The model under review builds one solid part; all positions refer to its coordinate system, in mm. A direction names the side the tool comes from. Give positions to 0.01 mm unless a question says otherwise; leave off trailing zeros. Order: outer loops, then holes, each group sorted by start corner. A loop starts at its lowest first (then second) coordinate and runs counter-clockwise, first axis right, second up.
```python
from build123d import *

# Parameters (mm, degrees)
SKETCH_1_W      = 69.25
SKETCH_1_H      = 48.25
SKETCH_1_R      = 1.275
EXTRUDE_1_DEPTH = 2
FILLET_1_R      = 2


with BuildPart() as part:
    # 草图1 → 凸台-拉伸1 (new body)
    with BuildSketch(Plane.XY):
        Rectangle(SKETCH_1_W, SKETCH_1_H)
        with Locations((-31.5, 21)):
            Circle(SKETCH_1_R, mode=Mode.SUBTRACT)
        with Locations((31.5, 21)):
            Circle(SKETCH_1_R, mode=Mode.SUBTRACT)
        with Locations((-31.5, -21)):
            Circle(SKETCH_1_R, mode=Mode.SUBTRACT)
        with Locations((31.5, -21)):
            Circle(SKETCH_1_R, mode=Mode.SUBTRACT)
        with BuildLine():
            Line((-16.5, 1.55), (-8.5, 1.55))
            ThreePointArc((-8.5, 1.55), (-6.95, 0), (-8.5, -1.55))
            Line((-8.5, -1.55), (-16.5, -1.55))
            ThreePointArc((-16.5, -1.55), (-18.05, 0), (-16.5, 1.55))
        make_face(mode=Mode.SUBTRACT)
        with BuildLine():
            Line((16.5, -1.55), (8.5, -1.55))
            ThreePointArc((8.5, -1.55), (6.95, 0), (8.5, 1.55))
            Line((8.5, 1.55), (16.5, 1.55))
            ThreePointArc((16.5, 1.55), (18.05, 0), (16.5, -1.55))
        make_face(mode=Mode.SUBTRACT)
    extrude(amount=EXTRUDE_1_DEPTH)

    # 圆角1
    fillet_1_edges = [part.edges().sort_by_distance(p)[0] for p in [
        (-34.625, 24.125, 1),
        (34.625, 24.125, 1),
        (34.625, -24.125, 1),
        (-34.625, -24.125, 1),
    ]]
    fillet(fillet_1_edges, radius=FILLET_1_R)


solid = part.part
```
1. Draft analysis for pull direction X (two halves, no side actions). For faces 1 (the cylindrical face through (30.226, -20.944, 0.986)), 2 (the flat face through (0, 0, 0)), 3 (the flat face through (34.625, 0, 1)), state which applies: pulls with the +X half, pulls with the -X half, needs draft (parallel to the pull), parting line crosses it, or undercut.
2. Take a section at C-C (z = 1.15). Write out the cut boundary in (x, y) (3 decimals).
3. To check wall thickness, follow line 1 (Y direction, x = 31.5, z = 1.5) (3 decimals); line 2 (Y direction, x = 9, z = 0.2) (3 decimals). State the ranges of each line that lie inside material, in increasing order.
4. Take a section at B-B (x = -31.5). Write out the cut boundary in (y, z) (3 decimals), and give its area (3 significant figures).
5. Take a section at A-A (y = -21). Write out the cut boundary in (x, z) (3 decimals).
6. For faces 4 (the cylindrical face through (-18.05, -0.03, 0.99)), 5 (the cylindrical face through (-34.055, 23.524, 1.014)), list the 3-axis set-ups (+Z, -Z, +X, -X, +Y, -Y) from which the entire face can be reached by the end or side of a thin tool; tool diameter is ignored.
7. Insertion check: pin 1 (2 mm diameter, centred on x = 31.5, y = 21, fed in from +Z). The pin has a flat end and moves straight along its axis. Give the tip position at first contact, or say it passes through.
Answer:
1. face 1: undercut
1. face 2: needs draft
1. face 3: pulls with the +X half
2. outline: (-34.625, -22.125) arc R2 ccw to (-32.625, -24.125) - (32.625, -24.125) arc R2 ccw to (34.625, -22.125) - (34.625, 22.125) arc R2 ccw to (32.625, 24.125) - (-32.625, 24.125) arc R2 ccw to (-34.625, 22.125) - close; hole circle Ø2.55 at (-31.5, -21); hole circle Ø2.55 at (-31.5, 21); hole (-16.5, -1.55) - (-8.5, -1.55) arc R1.55 ccw to (-8.5, 1.55) - (-16.5, 1.55) arc R1.55 ccw to start; hole (8.5, -1.55) - (16.5, -1.55) arc R1.55 ccw to (16.5, 1.55) - (8.5, 1.55) arc R1.55 ccw to start; hole circle Ø2.55 at (31.5, -21); hole circle Ø2.55 at (31.5, 21)
3. line 1: y = -24.125 to -22.275, -19.725 to 19.725, 22.275 to 24.125
3. line 2: y = -24.125 to -1.55, 1.55 to 24.125
4. outline: (-24.125, 0) - (-22.275, 0) - (-22.275, 2) - (-24.125, 2) - close; (-19.725, 0) - (19.725, 0) - (19.725, 2) - (-19.725, 2) - close; (22.275, 0) - (24.125, 0) - (24.125, 2) - (22.275, 2) - close
4. area: 86.3 mm2
5. outline: (-34.625, 0) - (-32.775, 0) - (-32.775, 2) - (-34.625, 2) - close; (-30.225, 0) - (30.225, 0) - (30.225, 2) - (-30.225, 2) - close; (32.775, 0) - (34.625, 0) - (34.625, 2) - (32.775, 2) - close
6. face 4: +Z, -Z
6. face 5: +Z, -Z, -X, +Y
7. pin 1: passes through
